CAD build for the part. Positions are in the model's coordinates, mm. Face numbers are marked on the shaded views. A direction names the side the tool comes from. Coordinates: 2 decimals unless noted, no trailing zeros. Write each loop counter-clockwise with the first axis right and the second up, starting at its lowest first coordinate (ties: lowest second). Pieces come first, ordered by that corner, then holes. Notation, with made-up numbers: M -11,17 L 6,17 A20 ccw 6,55 Z; hole C 43.5,27 d9. An arc over 180 degrees is marked long. Put each result on its own line as item: value. Start each with the question number.
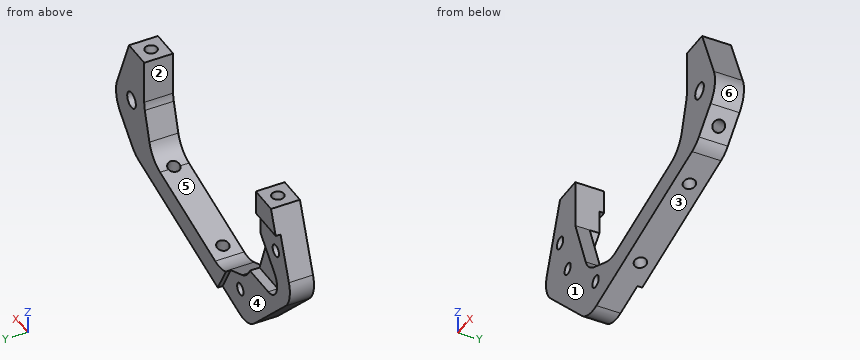
```python
from build123d import *

# Parameters (mm, degrees)
AUFSATZ_LINEAR_AUSTRAGEN1_DEPTH  = 6
VERRUNDUNG1_R                    = 6
DURCHGANGSLOCH_F_R_M21_OUTLINE_R = 1.2
DURCHGANGSLOCH_F_R_M21_DEPTH     = 6
SCHNITT_LINEAR_AUSTRAGEN1_DEPTH  = 3
SCHNITT_LINEAR_AUSTRAGEN2_DEPTH  = 1
M3_GEWINDEBOHRUNG2_D             = 2.5
M3_GEWINDEBOHRUNG3_D             = 2.5
M3_GEWINDEBOHRUNG3_DEPTH         = 6.5
M3_GEWINDEBOHRUNG3_TIP           = 0.751075774
M3_GEWINDEBOHRUNG4_D             = 2.5
M3_GEWINDEBOHRUNG4_DEPTH         = 6.5
M3_GEWINDEBOHRUNG4_TIP           = 0.751075774
DURCHGANGSLOCH_F_R_M32_OUTLINE_R = 1.7
DURCHGANGSLOCH_F_R_M32_DEPTH     = 6


# Read off the part's stored shape, not the designer's step: Durchgangsloch für M21, M3 Gewindebohrung1, Durchgangsloch für M32
with BuildPart() as part:
    # Skizze1 → Aufsatz-Linear austragen1 (new body)
    with BuildSketch(Plane(origin=(0, 0, 0), x_dir=(1, 0, 0), z_dir=(0, 1, 0))):
        Polygon((-6, 0), (0, 0), (0, 10), (5, 23.583657959), (14, 27.412076366), (41, 20.17744817), (44, 10), (44, 0), (50, 0), (56.190026492, 15), (47.606368533, 23.583657959), (5, 35), (-12.5, 17.5), align=None)
    extrude(amount=AUFSATZ_LINEAR_AUSTRAGEN1_DEPTH)

    # Verrundung1
    verrundung1_edges = [part.edges().sort_by_distance(p)[0] for p in [
        (-12.5, 3, -17.5),
        (5, 3, -35),
        (47.606368533, 3, -23.583657959),
        (56.190026492, 3, -15),
        (44, 3, -10),
        (41, 3, -20.17744817),
        (14, 3, -27.412076366),
        (5, 3, -23.583657959),
    ]]
    fillet(verrundung1_edges, radius=VERRUNDUNG1_R)

    # Durchgangsloch für M21 outline → Durchgangsloch für M21 (cut)
    with BuildSketch(Plane(origin=(0, 0, 0), x_dir=(1, 0, 0), z_dir=(0, 1, 0))):
        with Locations((-3, 18)):
            Circle(DURCHGANGSLOCH_F_R_M21_OUTLINE_R)
    extrude(amount=DURCHGANGSLOCH_F_R_M21_DEPTH, mode=Mode.SUBTRACT)

    # M3 Gewindebohrung1 outline → M3 Gewindebohrung1 (revolve, cut)
    with BuildSketch(Plane(origin=(47, 3, 0), x_dir=(1, 0, 0), z_dir=(0, -1, 0))):
        Polygon((0, 0), (0, -7.251075774), (1.25, -6.5), (1.25, 0), align=None)
    revolve(axis=Axis((47, 3, 0), (0, 0, 1)), mode=Mode.SUBTRACT)

    # M3 Gewindebohrung1 2 outline → M3 Gewindebohrung1 2 (revolve, cut)
    with BuildSketch(Plane(origin=(-3, 3, 0), x_dir=(1, 0, 0), z_dir=(0, -1, 0))):
        Polygon((0, 0), (0, -7.251075774), (1.25, -6.5), (1.25, 0), align=None)
    revolve(axis=Axis((-3, 3, 0), (0, 0, 1)), mode=Mode.SUBTRACT)

    # Skizze8 → Schnitt-Linear austragen1 (cut)
    with BuildSketch(Plane(origin=(0, 6, 0), x_dir=(1, 0, 0), z_dir=(0, 1, 0))):
        with BuildLine():
            Line((-5.48614249, 15.536446566), (0, 10))
            Line((0, 10), (4.293633921, 21.5))
            Line((4.293633921, 21.5), (-3, 21.5))
            ThreePointArc((-3, 21.5), (-6.23051366, 19.346767052), (-5.48614249, 15.536446566))
        make_face()
    extrude(amount=-SCHNITT_LINEAR_AUSTRAGEN1_DEPTH, mode=Mode.SUBTRACT)

    # Skizze9 → Schnitt-Linear austragen2 (cut)
    with BuildSketch(Plane(origin=(0, 6, 0), x_dir=(1, 0, 0), z_dir=(0, 1, 0))):
        Polygon((-7.857142857, 5), (0, 5), (15, 32.320508076), (5, 35), (-12.5, 17.5), align=None)
    extrude(amount=-SCHNITT_LINEAR_AUSTRAGEN2_DEPTH, mode=Mode.SUBTRACT)

    # M3 Gewindebohrung2 (through all)
    with Locations(Plane(origin=(0, 5, 0), x_dir=(1, 0, 0), z_dir=(0, 1, 0))):
        with Locations((8, 28.320508076), (-6, 10)):
            Hole(M3_GEWINDEBOHRUNG2_D / 2)

    # M3 Gewindebohrung3
    with Locations(Plane(origin=(9.084936491, 0, -33.905444566), x_dir=(-0.9659258262890604, 0, -0.2588190451025504), z_dir=(0.2588190451025504, 0, -0.9659258262890604))):
        with Locations((-31.272625875, 3), (-11.272625875, 3)):
            Hole(M3_GEWINDEBOHRUNG3_D / 2, depth=M3_GEWINDEBOHRUNG3_DEPTH)
            with Locations((0, 0, -(M3_GEWINDEBOHRUNG3_DEPTH + M3_GEWINDEBOHRUNG3_TIP / 2))):  # 118° drill point
                Cone(0, M3_GEWINDEBOHRUNG3_D / 2, M3_GEWINDEBOHRUNG3_TIP, mode=Mode.SUBTRACT)

    # M3 Gewindebohrung4
    with Locations(Plane(origin=(35.595013246, 0, -35.595013246), x_dir=(-0.7071067811865515, 0, -0.7071067811865436), z_dir=(0.7071067811865436, 0, -0.7071067811865515))):
        with Locations((-21.594316704, 3)):
            Hole(M3_GEWINDEBOHRUNG4_D / 2, depth=M3_GEWINDEBOHRUNG4_DEPTH)
            with Locations((0, 0, -(M3_GEWINDEBOHRUNG4_DEPTH + M3_GEWINDEBOHRUNG4_TIP / 2))):  # 118° drill point
                Cone(0, M3_GEWINDEBOHRUNG4_D / 2, M3_GEWINDEBOHRUNG4_TIP, mode=Mode.SUBTRACT)

    # Durchgangsloch für M32 outline → Durchgangsloch für M32 (cut)
    with BuildSketch(Plane(origin=(0, 0, 0), x_dir=(1, 0, 0), z_dir=(0, 1, 0))):
        with Locations((49, 12)):
            Circle(DURCHGANGSLOCH_F_R_M32_OUTLINE_R)
    extrude(amount=DURCHGANGSLOCH_F_R_M32_DEPTH, mode=Mode.SUBTRACT)


solid = part.part
```
(1) Slice it at B-B, the plane z = -8. Write the cut outline in (x, y), then the cut area to 3 significant figures.
(2) Slice it at A-A, the plane z = -12. Write the cut outline in (x, y).
(3) Two-plate mould, pull along X, no slides. Class the marked faces 1, 2 and 3: +X half, -X half, draft (parallel to the pull), parting line (faces both ways), or undercut.
(4) Drop flat-ended pins along their axis: pin 1 (5 mm diameter, centred on x = 8, z = -24, fed in from +Y); pin 2 (2 mm diameter, centred on x = -3, z = -18, fed in from +Y); pin 3 (1.5 mm diameter, centred on x = 47, y = 3, fed in from -Z); pin 4 (3 mm diameter, centred on y = 2, z = -6, fed in from +X) (3 decimals). Give the stop position or say it passes through.
(5) Which spindle directions (+Z, -Z, +X, -X, +Y, -Y) get a long thin tool onto all of the face, cutting with end or side? Do the marked faces 4, 5 and 6. Say none if no direction does.
(6) Drill centre lines: line 1 (X direction, y = 2.75, z = -2); line 2 (X direction, y = 3.8, z = -12); line 3 (Y direction, x = 47, z = -4). Where is each one in solid material? Low to high. Write a range as [from, to].
Result set:
1. outline: M -8.97,0 L 0,0 L 0,5 L -8.97,5 Z; M 44,0 L 53.3,0 L 53.3,6 L 44,6 Z
1. area: 101 mm^2
2. outline: M -10.46,0 L 0.74,0 L 0.74,3 L -1.98,3 L -1.98,5 L -10.46,5 Z; M 43.41,0 L 47.3,0 L 47.3,6 L 43.41,6 Z; M 50.7,0 L 54.9,0 L 54.9,6 L 50.7,6 Z
3. face 1: draft
3. face 2: undercut
3. face 3: +X half
4. pin 1: stops at y = 5
4. pin 2: passes through
4. pin 3: stops at z = -23.94
4. pin 4: stops at x = 53.095
5. face 4: -Z, -X, +Y
5. face 5: +Z, +Y, -Y
5. face 6: +X, +Y, -Y
6. line 1: x = [-6.74, -4.22], [-1.78, 0], [44, 45.78], [48.22, 50.83]
6. line 2: x = [-10.46, -1.98], [43.41, 47.3], [50.7, 54.9]
6. line 3: y = [0, 1.75], [4.25, 6]
